The model under review builds one solid part; all positions refer to its coordinate system, in mm. Face numbers are marked on the shaded views. Coordinates: 2 decimals unless noted, no trailing zeros. Order: outer loops, then holes, each group sorted by start corner. A loop starts at its lowest first (then second) coordinate and runs counter-clockwise, first axis right, second up. Notation, with made-up numbers: (55.5, -34) -> (105.5, -34) arc R24 ccw to (105.5, 1) -> close; hole circle Ø10 at (10, -19). An arc over 180 degrees is marked (long way). Put each result on its own line as item: value.
from build123d import *

# Parameters (mm, degrees)
ESTRUSIONE_SOTTILE1_DEPTH = 50
SCHIZZO4_R                = 6.5
TAGLIO_ESTRUSIONE1_DEPTH  = 144.603621124
SCHIZZO5_R                = 9
TAGLIO_ESTRUSIONE2_DEPTH  = 144.694119573
NERVATURA2_REACH          = 163.957
SCHIZZO6_WALL_W           = 354.197839966
SCHIZZO6_WALL_H           = 5


with BuildPart() as part:
    # Schizzo2 → Estrusione-Sottile1 (new, symmetric)
    with BuildSketch(Plane(origin=(0, 0, 0), x_dir=(0, 0, -1), z_dir=(1, 0, 0))):
        with BuildLine():
            Line((0, 102), (0, 16))
            ThreePointArc((0, 16), (4.686291501, 4.686291501), (16, 0))
            Line((16, 0), (101, 0))
            Line((101, 0), (101, 13))
            Line((101, 13), (16, 13))
            ThreePointArc((16, 13), (13.878679656, 13.878679656), (13, 16))
            Line((13, 16), (13, 102))
            Line((13, 102), (0, 102))
        make_face()
    extrude(amount=ESTRUSIONE_SOTTILE1_DEPTH, both=True)

    # Schizzo4 → Taglio-Estrusione1 (cut, through all)
    with BuildSketch(Plane(origin=(0, 13, 0), x_dir=(1, 0, 0), z_dir=(0, 1, 0))):
        with Locations(Location((-25, 56, 0), (0, 0, 270))):
            Circle(SCHIZZO4_R)
        with Locations(Location((25, 56, 0), (0, 0, 270))):
            Circle(SCHIZZO4_R)
    extrude(amount=-TAGLIO_ESTRUSIONE1_DEPTH, mode=Mode.SUBTRACT)

    # Schizzo5 → Taglio-Estrusione2 (cut, through all)
    with BuildSketch(Plane(origin=(0, 0, -13), x_dir=(-1, 0, 0), z_dir=(0, 0, -1))):
        with Locations((0, 69)):
            Circle(SCHIZZO5_R)
    extrude(amount=-TAGLIO_ESTRUSIONE2_DEPTH, mode=Mode.SUBTRACT)

    # Schizzo6 wall → Nervatura2 (add, up to next)
    with BuildSketch(Plane(origin=(25, 23, -23), x_dir=(0, -0.707106781187, -0.707106781187), z_dir=(0, 0.707106781187, -0.707106781187)), mode=Mode.PRIVATE) as nervatura2_sk1:
        Rectangle(SCHIZZO6_WALL_W, SCHIZZO6_WALL_H)
    nervatura2_tool1 = extrude(nervatura2_sk1.sketch, amount=-NERVATURA2_REACH, mode=Mode.PRIVATE) - part.part
    nervatura2 = nervatura2_tool1.solids().sort_by_distance((25, 23, -23))[0]
    add(nervatura2)

    # Specchia1: Nervatura2 across plane
    add(nervatura2.mirror(Plane(origin=(0, 0, 0), x_dir=(0, 0, 1), z_dir=(1, 0, 0))))


solid = part.part
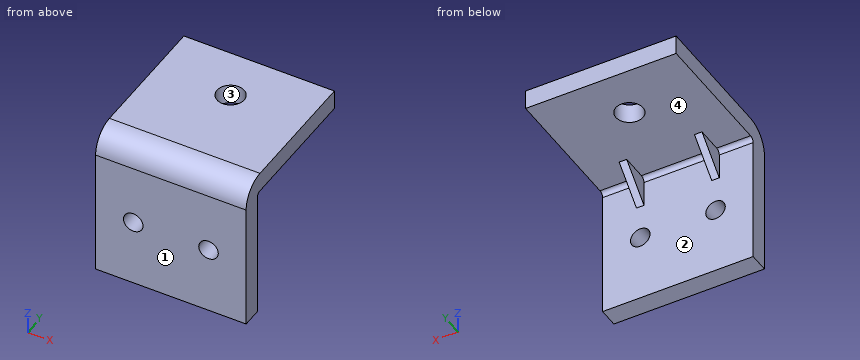
Item 1: Consider section B-B on z = -56. Write out the cut boundary in (x, y), and give its area (3 significant figures).
Answers below:
outline: (-50, 0) -> (-31.5, 0) -> (-31.5, 13) -> (-50, 13) -> close; (-18.5, 0) -> (18.5, 0) -> (18.5, 13) -> (-18.5, 13) -> close; (31.5, 0) -> (50, 0) -> (50, 13) -> (31.5, 13) -> close
area: 962 mm^2
Item 2: Mouldability with a two-part tool opening along Y and no side actions: class the marked faces 1, 2, 3 and 4 as +Y half, -Y half, draft (parallel to the pull), parting line (faces both ways), or undercut.
Answers below:
face 1: -Y half
face 2: +Y half
face 3: undercut
face 4: draft
Item 3: For line 1 (X direction, y = 10.75, z = -56); line 2 (Z direction, x = -18.5, y = 77.5); line 3 (X direction, y = 20, z = -20), list the stretches that pass through material, from the lowest coordinate up. Write a range as from..to.
Answers below:
line 1: -50..-31.5, -18.5..18.5, 31.5..50
line 2: -13..0
line 3: -27.5..-22.5, 22.5..27.5
Item 4: For pin 1 Ø5 at (x, y) = (2.5, 15) entering from -Z; pin 2 Ø10 at (y, z) = (22, -21.5) entering from -X; pin 3 Ø1.5 at (x, y) = (-31.5, 41) entering from -Z; pin 4 Ø10 at (y, z) = (22.5, -26) entering from +X, all flat-tipped, find the tip position at first contact; note any pin that passes through.
Answers below:
pin 1: z = -101
pin 2: x = -27.5
pin 3: z = -13
pin 4: x = 27.5
Item 5: Consider section D-D on x = 36. Write out the cut boundary in (y, z).
Answers below:
outline: (0, -101) -> (13, -101) -> (13, -16) arc R3 cw to (16, -13) -> (102, -13) -> (102, 0) -> (16, 0) arc R16 ccw to (0, -16) -> close
Item 6: Consider section C-C on y = 69. Write out the cut boundary in (x, z), and give its area (3 significant figures).
Answers below:
outline: (-50, -13) -> (-9, -13) -> (-9, 0) -> (-50, 0) -> close; (9, -13) -> (50, -13) -> (50, 0) -> (9, 0) -> close
area: 1,070 mm^2
Item 7: Consider section A-A on x = 0. Write out the cut boundary in (y, z).
Answers below:
outline: (0, -101) -> (13, -101) -> (13, -16) arc R3 cw to (16, -13) -> (60, -13) -> (60, 0) -> (16, 0) arc R16 ccw to (0, -16) -> close; (78, -13) -> (102, -13) -> (102, 0) -> (78, 0) -> close
